```python
from build123d import *

# Parameters (mm, degrees)
SKETCH_1_W      = 67
SKETCH_1_H      = 35
EXTRUDE_1_DEPTH = 56
EXTRUDE_START   = -11
EXTRUDE_2_DEPTH = 35
SKETCH_3_W      = 13.5
SKETCH_3_H      = 27
EXTRUDE_3_DEPTH = 0.6


with BuildPart() as part:
    # 草图1 → 拉伸1 (new body)
    with BuildSketch(Plane.XY):
        Rectangle(SKETCH_1_W, SKETCH_1_H)
    extrude(amount=EXTRUDE_1_DEPTH)

    # 草图2 → 拉伸2 (add)
    with BuildSketch(Plane.XY.offset(56).offset(EXTRUDE_START)):
        with BuildLine():
            Line((-12, 30), (12, 30))
            ThreePointArc((12, 30), (19.071067812, 27.071067812), (22, 20))
            Line((22, 20), (22, -20))
            ThreePointArc((22, -20), (19.071067812, -27.071067812), (12, -30))
            Line((12, -30), (-12, -30))
            ThreePointArc((-12, -30), (-19.071067812, -27.071067812), (-22, -20))
            Line((-22, -20), (-22, 20))
            ThreePointArc((-22, 20), (-19.071067812, 27.071067812), (-12, 30))
        make_face()
    extrude(amount=-EXTRUDE_2_DEPTH)

    # 草图3 → 拉伸3 (add)
    # profile 1 of 2: a face of its own
    with BuildSketch(Plane(origin=(0, 0, 0), x_dir=(-1, 0, 0), z_dir=(0, 0, -1))):
        with Locations((-40.25, 0)):
            Rectangle(SKETCH_3_W, SKETCH_3_H)
        with BuildLine():
            Line((-43, 2.25), (-39, 2.25))
            ThreePointArc((-39, 2.25), (-36.75, 0), (-39, -2.25))
            Line((-39, -2.25), (-43, -2.25))
            ThreePointArc((-43, -2.25), (-45.25, 0), (-43, 2.25))
        make_face(mode=Mode.SUBTRACT)
    # profile 2 of 2: a face of its own
    with BuildSketch(Plane(origin=(0, 0, 0), x_dir=(-1, 0, 0), z_dir=(0, 0, -1))):
        with Locations((40.25, 0)):
            Rectangle(SKETCH_3_W, SKETCH_3_H)
        with BuildLine():
            Line((43, 2.25), (39, 2.25))
            ThreePointArc((39, 2.25), (36.75, 0), (39, -2.25))
            Line((39, -2.25), (43, -2.25))
            ThreePointArc((43, -2.25), (45.25, 0), (43, 2.25))
        make_face(mode=Mode.SUBTRACT)
    extrude(amount=-EXTRUDE_3_DEPTH)


solid = part.part
```
Model file for the job. Use its own axes, mm. A direction names the side the tool comes from. Give positions to 0.01 mm unless a question says otherwise; leave off trailing zeros. Loops run counter-clockwise (first coordinate to the right, second up) from the corner with the lowest first, then second, coordinate; pieces in that order, holes last. Notation, with made-up numbers: (-10, -27.75) - (47, -27.75) arc R14 ccw to (47, -17.75) - close; hole circle Ø11 at (75.25, 11). An arc over 180 degrees is marked (long way). One line per item, written item: value. Start each with the question number.
1. Slice it at A-A (y = 0). List the corners of the cut face in (x, z), plus the area to 3 significant figures.
2. Slice it at C-C (z = 43). List the corners of the cut face in (x, y), plus the area to 3 significant figures.
3. Pull direction X, two halves, no side cores. Call faces 1 (the cylindrical face through (-36.75, 0.05, 0.3)), 2 (the flat face through (0, -24, 10)), 3 (the cylindrical face through (-19.15, 26.99, 27.74)): pulls with the +X half, pulls with the -X half, needs draft (parallel to the pull), parting line crosses it, or undercut.
4. Pin check, flat tips, straight feed: pin 1 (10 mm diameter, centred on x = 8.5, y = -24, fed in from -Z); pin 2 (11 mm diameter, centred on x = 43.5, y = 3, fed in from +Z); pin 3 (2 mm diameter, centred on y = -19, z = 26, fed in from -X). Stop position of each tip, or through.
5. Probe L1, parallel to X at y = 14, z = 14.5; L2, parallel to Y at x = 25.5, z = 37; L3, parallel to X at y = 21, z = 36.5. List the from-to ranges inside material, lowest first. Write a range as from..to.
6. Which spindle directions (+Z, -Z, +X, -X, +Y, -Y) get a long thin tool onto all of the face, cutting with end or side? Do faces 4 (the flat face through (0, 24, 45)), 5 (the cylindrical face through (36.75, 0.05, 0.3)), 6 (the flat face through (-22, -19, 28)). Say none if no direction does.
7. Slice it at B-B (y = -12). List the corners of the cut face in (x, z).
8. Slice it at D-D (x = 8.5). List the corners of the cut face in (y, z), plus the area to 4 significant figures.
Solution:
1. outline: (-47, 0) - (-45.25, 0) - (-45.25, 0.6) - (-47, 0.6) - close; (-36.75, 0) - (36.75, 0) - (36.75, 0.6) - (33.5, 0.6) - (33.5, 56) - (-33.5, 56) - (-33.5, 0.6) - (-36.75, 0.6) - close; (45.25, 0) - (47, 0) - (47, 0.6) - (45.25, 0.6) - close
1. area: 3,760 mm^2
2. outline: (-33.5, -17.5) - (-22, -17.5) - (-22, -20) arc R10 ccw to (-12, -30) - (12, -30) arc R10 ccw to (22, -20) - (22, -17.5) - (33.5, -17.5) - (33.5, 17.5) - (22, 17.5) - (22, 20) arc R10 ccw to (12, 30) - (-12, 30) arc R10 ccw to (-22, 20) - (-22, 17.5) - (-33.5, 17.5) - close
2. area: 3,360 mm^2
3. face 1: undercut
3. face 2: needs draft
3. face 3: pulls with the -X half
4. pin 1: stops at z = 10
4. pin 2: stops at z = 0.6
4. pin 3: stops at x = -22
5. L1: x = -33.5..33.5
5. L2: y = -17.5..17.5
5. L3: x = -21.95..21.95
6. face 4: +Z, +X, -X, +Y
6. face 5: +Z, -Z
6. face 6: +Z, -Z, -X, -Y
7. outline: (-47, 0) - (47, 0) - (47, 0.6) - (33.5, 0.6) - (33.5, 56) - (-33.5, 56) - (-33.5, 0.6) - (-47, 0.6) - close
8. outline: (-30, 10) - (-17.5, 10) - (-17.5, 0) - (17.5, 0) - (17.5, 10) - (30, 10) - (30, 45) - (17.5, 45) - (17.5, 56) - (-17.5, 56) - (-17.5, 45) - (-30, 45) - close
8. area: 2,835 mm^2
